Autodesk Inventor part; units mm, degrees
ref_plane "YZ Plane" through (0, 0, 0) normal (1, 0, 0) x (0, 1, 0)
ref_plane "XZ Plane" through (0, 0, 0) normal (0, 1, 0) x (-1, 0, 0)
ref_plane "XY Plane" through (0, 0, 0) normal (0, 0, 1) x (1, 0, 0)
sketch "Sketch1" plane through (0, 0, 0) normal (0, 0, 1) x (1, 0, 0)
  line L0 (0, 0) -> (0, 4438.8737)
  line L1 (0, 4438.8737) -> (100, 4438.8737)
  line L2 (100, 4438.8737) -> (200, 0)
  line L3 (200, 0) -> (0, 0)
  circle A0 centre (0, 0) radius 30
  line L4 (0, 1479.6246) -> (166.6667, 1479.6246)
  line L5 (0, 2959.2492) -> (133.3333, 2959.2492)
  circle A1 centre (0, 1479.6246) radius 30
  circle A2 centre (0, 2959.2492) radius 30
  line L6 (190.8761, 405) -> (120.8761, 405)
  line L7 (120.8761, 405) -> (120.8761, 410)
  line L8 (120.8761, 410) -> (190.8761, 410)
  line L9 (190.8761, 410) -> (190.8761, 405)
  line L10 (109.6148, 909.8732) -> (179.6148, 909.8732)
  line L11 (179.6148, 904.8732) -> (109.6148, 904.8732)
  line L12 (109.6148, 904.8732) -> (109.6148, 909.8732)
  line L13 (179.6148, 909.8732) -> (179.6148, 904.8732)
  line L14 (98.3535, 1409.7463) -> (168.3535, 1409.7463)
  line L15 (168.3535, 1404.7463) -> (98.3535, 1404.7463)
  line L16 (98.3535, 1404.7463) -> (98.3535, 1409.7463)
  line L17 (168.3535, 1409.7463) -> (168.3535, 1404.7463)
  line L18 (87.0923, 1909.6195) -> (157.0923, 1909.6195)
  line L19 (157.0923, 1904.6195) -> (87.0923, 1904.6195)
  line L20 (87.0923, 1904.6195) -> (87.0923, 1909.6195)
  line L21 (157.0923, 1909.6195) -> (157.0923, 1904.6195)
  line L22 (75.831, 2409.4927) -> (145.831, 2409.4927)
  line L23 (145.831, 2404.4927) -> (75.831, 2404.4927)
  line L24 (75.831, 2404.4927) -> (75.831, 2409.4927)
  line L25 (145.831, 2409.4927) -> (145.831, 2404.4927)
  line L26 (64.5698, 2909.3658) -> (134.5698, 2909.3658)
  line L27 (134.5698, 2904.3658) -> (64.5698, 2904.3658)
  line L28 (64.5698, 2904.3658) -> (64.5698, 2909.3658)
  line L29 (134.5698, 2909.3658) -> (134.5698, 2904.3658)
  line L30 (53.3085, 3409.239) -> (123.3085, 3409.239)
  line L31 (123.3085, 3404.239) -> (53.3085, 3404.239)
  line L32 (53.3085, 3404.239) -> (53.3085, 3409.239)
  line L33 (123.3085, 3409.239) -> (123.3085, 3404.239)
  line L34 (42.0472, 3909.1122) -> (112.0472, 3909.1122)
  line L35 (112.0472, 3904.1122) -> (42.0472, 3904.1122)
  line L36 (42.0472, 3904.1122) -> (42.0472, 3909.1122)
  line L37 (112.0472, 3909.1122) -> (112.0472, 3904.1122)
  line L38 (0, 1629.6246) -> (163.2874, 1629.6246)
  line L39 (0, 3079.2492) -> (130.6299, 3079.2492)
  circle A3 centre (20, 1609.6246) radius 9
  circle A4 centre (150.0408, 1329.6246) radius 9
  circle A5 centre (173.2365, 300) radius 9
  line L40 (173.2365, 300) -> (150.0408, 1329.6246)
  point P0 (30, 2959.2492)
  point P1 (0, 2929.2492)
  point P2 (0, 1509.6246)
  point P3 (0, 1449.6246)
  point P4 (0, 30)
  point P5 (30, 0)
  point P6 (190.7634, 410)
  point P7 (179.5022, 909.8732)
  point P8 (168.3535, 1404.7463)
  point P9 (168.2409, 1409.7463)
  point P10 (30, 1479.6246)
  dimension "d65" = 100
  dimension "d67" = 200
  dimension "d68" = 60
  dimension "d69" = 1480
  dimension "d70" = 1480
  dimension "d71" = 1480
  dimension "d72" = 5
  dimension "d73" = 70
  dimension "d74" = 410
  dimension "d77" = 500
  dimension "d82" = 120
  dimension "d83" = 150
  dimension "d88" = 20
  dimension "d89" = 20
  dimension "d90" = 18
  dimension "d91" = 20
  dimension "d92" = 300
  dimension "d93" = 300
extrude "Plate3" add sketch "Sketch1" along normal blind 4 contours L38 L2 L4 A1 L0 | L4 L2 L14 L16 L15 L10 L12 L11 L40 L8 L7 L6 L3 A0 L0 A1 | L2 L8 L40 L11
chamfer "Corner Chamfer2" distance 3 angle 45 6 edges at (190.7634, 410, 2) (190.8761, 405, 2) (179.6148, 904.8732, 2) (179.5022, 909.8732, 2) (168.3535, 1404.7463, 2) (168.2409, 1409.7463, 2)
equation "\"BendRadius\" = Thickness"
equation "\"BendReliefWidth\" = Thickness"
equation "\"BendReliefDepth\" = 0.5 * Thickness"
equation "\"CornerReliefSize\" = 4 * Thickness"
equation "\"MinimumRemnant\" = 2 * Thickness"
equation "\"TransitionRadius\" = BendRadius"
equation "\"JacobiRadiusSize\" = BendRadius"
equation "\"GapSize\" = Thickness"
properties part number "GBK 3112 central main rib" material "Steel"
Here's how the part is built. I have some questions about the finished solid (model axes, mm). Coordinates: 2 decimals unless noted, no trailing zeros. Write each loop counter-clockwise with the first axis right and the second up, starting at its lowest first coordinate (ties: lowest second). Pieces come first, ordered by that corner, then holes.
Item 1: I want a section at B-B on y = 524. Write out the boundary of the cut face in (x, z), and give its area (3 significant figures).
Item 2: If I drill on line 1 (Y direction, x = 125, z = 2.3); line 2 (Y direction, x = 20, z = 2.2); line 3 (X direction, y = 794.5, z = 1.15), over which ranges is the centre line in solid material (lowest first)?
Item 3: I want a section at A-A on z = 3.35. Write out the boundary of the cut face in (x, y).
Item 4: I want a section at C-C on y = 1356. Write out the boundary of the cut face in (x, z), and give its area (3 significant figures).
Item 5: Will these pins go through, and if not, where does the flat tip stop? pin 1 (2 mm diameter, centred on y = 214, z = 2.5, fed in from -X); pin 2 (1 mm diameter, centred on y = 1228, z = 3, fed in from +X); pin 3 (2 mm diameter, centred on y = 1407, z = 2.5, fed in from +X); pin 4 (1.5 mm diameter, centred on y = 214.5, z = 3.5, fed in from +X).
Findings below:
1. outline: (0, 0) - (188.2, 0) - (188.2, 4) - (0, 4) - close
1. area: 753 mm2
2. line 1: y = 0 to 405, 410 to 904.87, 909.87 to 1404.75, 1409.75 to 1629.62
2. line 2: y = 22.36 to 1457.26, 1501.99 to 1600.62, 1618.62 to 1629.62
2. line 3: x = 0 to 182.1
3. outline: (0, 30) arc R30 cw to (30, 0) - (200, 0) - (190.94, 402) - (187.88, 405) - (120.88, 405) - (120.88, 410) - (187.76, 410) - (190.7, 413) - (179.68, 901.87) - (176.61, 904.87) - (109.61, 904.87) - (109.61, 909.87) - (176.5, 909.87) - (179.43, 912.87) - (168.42, 1401.75) - (165.35, 1404.75) - (98.35, 1404.75) - (98.35, 1409.75) - (165.24, 1409.75) - (168.17, 1412.75) - (163.29, 1629.62) - (0, 1629.62) - (0, 1509.62) arc R30 cw to (0, 1449.62) - close; hole circle Ø18 at (20, 1609.62); hole circle Ø18 at (150.04, 1329.62); hole circle Ø18 at (173.24, 300)
4. outline: (0, 0) - (169.45, 0) - (169.45, 4) - (0, 4) - close
4. area: 678 mm2
5. pin 1: stops at x = 0
5. pin 2: stops at x = 172.35
5. pin 3: stops at x = 98.35
5. pin 4: stops at x = 195.18
